Could you check a few things on this model? Use its own coordinates, in mm. A direction names the side the tool comes from. Give positions to 0.01 mm unless a question says otherwise; leave off trailing zeros. Order: outer loops, then holes, each group sorted by start corner. A loop starts at its lowest first (then second) coordinate and runs counter-clockwise, first axis right, second up. Notation, with made-up numbers: (35.5, -4.5) -> (59.5, -4.5) arc R25 ccw to (59.5, 19.5) -> close; hole circle Ø4 at (23.25, 80). An arc over 180 degrees is marked (long way). Write each question's results on one line, items separated by ' | '.
```python
from build123d import *

# Parameters (mm, degrees)
PAD026_DEPTH  = 12
SKETCH071_R   = 20
SKETCH071_R_2 = 13
PAD027_DEPTH  = 10


with BuildPart() as part:
    # Sketch070 (on Face5 of Binder016) → Pad026 (new body)
    with BuildSketch(Plane.XY.offset(8)):
        with BuildLine():
            ThreePointArc((-12.5, -3.570714), (0, -13), (12.5, -3.570714))
            Line((12.5, -11.521719), (12.5, -3.570714))
            ThreePointArc((-12.5, -11.521719), (0, -17), (12.5, -11.521719))
            Line((-12.5, -11.521719), (-12.5, -3.570714))
        make_face()
    pad026 = extrude(amount=PAD026_DEPTH)

    # Mirrored: Pad026 across XZ
    add(pad026.mirror(Plane.XZ))

    # Sketch071 (on Face4 of Mirrored) → Pad027 (join)
    with BuildSketch(Plane.XY.offset(20)):
        Circle(SKETCH071_R)
        Circle(SKETCH071_R_2, mode=Mode.SUBTRACT)
    extrude(amount=PAD027_DEPTH)

    # Mirrored001: Pad026 across XZ
    add(pad026.mirror(Plane.XZ))


solid = part.part
```
Q1. I'm going to push flat-ended pins straight in: pin 1 Ø8.5 at (y, z) = (7.5, 13) entering from -X; pin 2 Ø2 at (y, z) = (15, 13) entering from +X; pin 3 Ø10 at (y, z) = (-15, 25) entering from -X. Where does each tip first touch, or does it pass through?
Here are the results:
pin 1: stops at x = -12.5 | pin 2: stops at x = 9.64 | pin 3: stops at x = -17.32
Q2. For faces 1 (the cylindrical face through (0, 17, 14)), 2 (the flat face through (-12.5, -8, 14)), 3 (the flat face through (0.2, 13.2, 8)), 4 (the cylindrical face through (0, -17, 14)), 5 (the flat face through (12.5, 8, 14)), which set-ups out of +Z, -Z, +X, -X, +Y, -Y let a thin tool reach every point of the face, with its end or its side?
Here are the results:
face 1: -Z, +Y | face 2: -Z, -X, +Y, -Y | face 3: -Z, +X, -X, +Y, -Y | face 4: -Z, -Y | face 5: -Z, +X, +Y, -Y
Q3. Suppose I cut it at D-D on z = 27.5. Please give me the cut outline in (x, y).
Here are the results:
outline: circle Ø40 at (0, 0); hole circle Ø26 at (0, 0)
Q4. I need wall thicknesses on line 1 along Y through (x, z) = (0, 24.25); line 2 along Z through (x, y) = (-9, 16); line 3 along Y through (x, z) = (4, 19.5). Which ranges of each line are inside material? Lowest first, please.
Here are the results:
line 1: y = -20 to -13, 13 to 20 | line 2: z = 20 to 30 | line 3: y = -16.52 to -12.37, 12.37 to 16.52
Q5. Suppose I cut it at A-A on x = 0. Please give me the cut outline in (y, z), and give its area (3 significant figures).
Here are the results:
outline: (-20, 20) -> (-17, 20) -> (-17, 8) -> (-13, 8) -> (-13, 30) -> (-20, 30) -> close; (13, 8) -> (17, 8) -> (17, 20) -> (20, 20) -> (20, 30) -> (13, 30) -> close | area: 236 mm²
Q6. Suppose I cut it at B-B on z = 11.25. Please give me the cut outline in (x, y).
Here are the results:
outline: (-12.5, -11.52) arc R17 ccw to (12.5, -11.52) -> (12.5, -3.57) arc R13 cw to (-12.5, -3.57) -> close; (-12.5, 3.57) arc R13 cw to (12.5, 3.57) -> (12.5, 11.52) arc R17 ccw to (-12.5, 11.52) -> close
Q7. Suppose I cut it at C-C on y = 10. Please give me the cut outline in (x, z).
Here are the results:
outline: (-17.32, 20) -> (-12.5, 20) -> (-12.5, 8) -> (-8.31, 8) -> (-8.31, 30) -> (-17.32, 30) -> close; (8.31, 8) -> (12.5, 8) -> (12.5, 20) -> (17.32, 20) -> (17.32, 30) -> (8.31, 30) -> close
